```python
from build123d import *

# Parameters (mm, degrees)
SKETCH1_W           = 125
SKETCH1_H           = 30
BOSS_EXTRUDE1_DEPTH = 7
SKETCH2_R           = 2
CUT_EXTRUDE1_DEPTH  = 10


with BuildPart() as part:
    # Sketch1 → Boss-Extrude1 (new body)
    with BuildSketch(Plane(origin=(0, 0, 0), x_dir=(1, 0, 0), z_dir=(0, 1, 0))):
        with Locations((-40.010460251, 50.167364017)):
            Rectangle(SKETCH1_W, SKETCH1_H)
    extrude(amount=BOSS_EXTRUDE1_DEPTH)

    # Sketch2 → Cut-Extrude1 (cut)
    with BuildSketch(Plane.XZ):
        with Locations((-70.260460251, -61.167364017)):
            Circle(SKETCH2_R)
        with Locations((-41.010460251, -61.167364017)):
            Circle(SKETCH2_R)
        with Locations((-11.760460251, -61.167364017)):
            Circle(SKETCH2_R)
    extrude(amount=-CUT_EXTRUDE1_DEPTH, mode=Mode.SUBTRACT)


solid = part.part
```
The model under review builds one solid part; all positions refer to its coordinate system, in mm. Round coordinates to 2 decimals unless told otherwise and drop trailing zeros. Loops run counter-clockwise (first coordinate to the right, second up) from the corner with the lowest first, then second, coordinate; pieces in that order, holes last.
1) Consider section A-A on x = -71. State the section outline as (y, z) points, then the cut area to 3 significant figures.
Values follow:
outline: (0, -65.17) - (7, -65.17) - (7, -63.03) - (0, -63.03) - close; (0, -59.31) - (7, -59.31) - (7, -35.17) - (0, -35.17) - close
area: 184 mm2
2) The part is to be moulded in two halves that separate along X. For faces 1 (the face through (-43.01, 3.45, -61.08)), 2 (the face through (22.49, 3, -50)), 3 (the face through (-41, 3, -35.167)), say which applies: pulls with the +X half, pulls with the -X half, needs draft (parallel to the pull), parting line crosses it, or undercut.
Values follow:
face 1: undercut
face 2: pulls with the +X half
face 3: needs draft
3) Clearance check with flat-ended pins moving along their axes: P1, Ø3, axis at x = -11.76, z = -61.17, coming from the +Y side; P2, Ø1.5, axis at x = -11, z = -59, coming from the -Y side. State where each tip first meets the part, or that it passes through.
Values follow:
P1: passes through
P2: stops at y = 0
4) Wall thickness on line 1 along X through (y, z) = (6.25, -61.75); line 2 along Z through (x, y) = (-10.5, 1.25): over which ranges is each line inside the solid? List them lowest first.
Values follow:
line 1: x = -102.51 to -72.17, -68.35 to -42.92, -39.1 to -13.67, -9.85 to 22.49
line 2: z = -65.17 to -62.72, -59.61 to -35.17
